```python
from build123d import *

# Parameters (mm, degrees)
F7_W      = 30
F7_H      = 30
F8_DEPTH  = 1700
F15_DEPTH = 15
F17_DEPTH = 15
F19_DEPTH = 15
F21_DEPTH = 15


with BuildPart() as f8:
    # F7 (on Top) → F8 (new body)
    with BuildSketch(Plane.XY):
        with Locations((-500, -15)):
            Rectangle(F7_W, F7_H)
    extrude(amount=F8_DEPTH)



with BuildPart() as f8b:
    # F7 (on Top) → F8, piece 2 (new body)
    with BuildSketch(Plane.XY):
        with Locations((500, -15)):
            Rectangle(F7_W, F7_H)
    extrude(amount=F8_DEPTH)


with BuildPart() as f8_1:
    add(f8.part)

    add(f8b.part)  # F15 merges F8b
    # F14 (on offset) → F15 (join)
    with BuildSketch(Plane.XY.offset(450)):
        with BuildLine():
            Line((485, 0), (0, 0))
            Line((0, 0), (-485, 0))
            Line((-485, 0), (-485, -30))
            Line((-485, -30), (-515, -30))
            Line((-515, -30), (-515, 0))
            Line((-515, 0), (-650, 0))
            Line((-650, 0), (-650, -360))
            ThreePointArc((-650, -360), (-638.2842712475, -388.2842712475), (-610, -400))
            Line((-610, -400), (0, -400))
            Line((0, -400), (610, -400))
            ThreePointArc((610, -400), (638.2842712475, -388.2842712475), (650, -360))
            Line((650, -360), (650, 0))
            Line((650, 0), (515, 0))
            Line((515, 0), (515, -30))
            Line((515, -30), (485, -30))
            Line((485, -30), (485, 0))
        make_face()
    extrude(amount=-F15_DEPTH)

    # F16 (on offset) → F17 (join)
    with BuildSketch(Plane.XY.offset(750)):
        with BuildLine():
            Line((0, -400), (610, -400))
            ThreePointArc((610, -400), (638.2842712475, -388.2842712475), (650, -360))
            Line((650, -360), (650, 0))
            Line((650, 0), (515, 0))
            Line((515, 0), (515, -30))
            Line((515, -30), (485, -30))
            Line((485, -30), (485, 0))
            Line((485, 0), (0, 0))
            Line((0, 0), (-485, 0))
            Line((-485, 0), (-485, -30))
            Line((-485, -30), (-515, -30))
            Line((-515, -30), (-515, 0))
            Line((-515, 0), (-650, 0))
            Line((-650, 0), (-650, -360))
            ThreePointArc((-650, -360), (-638.2842712475, -388.2842712475), (-610, -400))
            Line((-610, -400), (0, -400))
        make_face()
    extrude(amount=-F17_DEPTH)

    # F18 (on offset) → F19 (join)
    with BuildSketch(Plane.XY.offset(1150)):
        with BuildLine():
            Line((0, -400), (610, -400))
            ThreePointArc((610, -400), (638.2842712475, -388.2842712475), (650, -360))
            Line((650, -360), (650, 0))
            Line((650, 0), (515, 0))
            Line((515, 0), (515, -30))
            Line((515, -30), (485, -30))
            Line((485, -30), (485, 0))
            Line((485, 0), (0, 0))
            Line((0, 0), (-485, 0))
            Line((-485, 0), (-485, -30))
            Line((-485, -30), (-515, -30))
            Line((-515, -30), (-515, 0))
            Line((-515, 0), (-650, 0))
            Line((-650, 0), (-650, -360))
            ThreePointArc((-650, -360), (-638.2842712475, -388.2842712475), (-610, -400))
            Line((-610, -400), (0, -400))
        make_face()
    extrude(amount=-F19_DEPTH)

    # F20 (on offset) → F21 (join)
    with BuildSketch(Plane.XY.offset(1550)):
        with BuildLine():
            Line((0, -400), (610, -400))
            ThreePointArc((610, -400), (638.2842712475, -388.2842712475), (650, -360))
            Line((650, -360), (650, 0))
            Line((650, 0), (515, 0))
            Line((515, 0), (515, -30))
            Line((515, -30), (485, -30))
            Line((485, -30), (485, 0))
            Line((485, 0), (0, 0))
            Line((0, 0), (-485, 0))
            Line((-485, 0), (-485, -30))
            Line((-485, -30), (-515, -30))
            Line((-515, -30), (-515, 0))
            Line((-515, 0), (-650, 0))
            Line((-650, 0), (-650, -360))
            ThreePointArc((-650, -360), (-638.2842712475, -388.2842712475), (-610, -400))
            Line((-610, -400), (0, -400))
        make_face()
    extrude(amount=-F21_DEPTH)


solid = f8_1.part
```
Geometry: final body of the model. Coordinates: model frame, mm. Give positions to 0.01 mm unless a question says otherwise; leave off trailing zeros. Order: outer loops, then holes, each group sorted by start corner. A loop starts at its lowest first (then second) coordinate and runs counter-clockwise, first axis right, second up. Notation, with made-up numbers: (33.25, 54) -> (38.25, 54) arc R16 ccw to (38.25, 62) -> close; hole circle Ø3 at (89, 34). An arc over 180 degrees is marked (long way). Write each question's results on one line, items separated by ' | '. Start each with the question number.
1) Section B-B (y = -97.5). Return loops of the section in (x, z).
2) Line query: line 1 (Z direction, x = -59, y = -298); line 2 (Y direction, x = -491.5, z = 1132.5). Output: solid intervals per line, ascending. Write a range as from..to.
3) Section A-A (x = -296). Return loops of the section in (y, z).
4) Section C-C (z = 1450.5). Return loops of the section in (x, y), then the cut area to 3 significant figures.
5) Draft query along Z for faces 1 (the flat face through (-9, -197, 1150)), 2 (the flat face through (-3, 0, 1539)). Return one class per face: pulls with the +Z half, pulls with the -Z half, needs draft (parallel to the pull), parting line crosses it, or undercut.
6) First-contact query: pin 1 (9 mm diameter, centred on y = -15.5, z = 271.5, fed in from +X); pin 2 (24 mm diameter, centred on x = 493, z = 525.5, fed in from -Y); pin 3 (9 mm diameter, centred on y = -11.5, z = 995.5, fed in from -X). Flat tips, straight axial feed; report the tip coordinate or a pass-through.
Calculated:
1) outline: (-650, 435) -> (650, 435) -> (650, 450) -> (-650, 450) -> close; (-650, 735) -> (650, 735) -> (650, 750) -> (-650, 750) -> close; (-650, 1135) -> (650, 1135) -> (650, 1150) -> (-650, 1150) -> close; (-650, 1535) -> (650, 1535) -> (650, 1550) -> (-650, 1550) -> close
2) line 1: 435..450, 735..750, 1135..1150, 1535..1550 | line 2: -30..0
3) outline: (-400, 435) -> (0, 435) -> (0, 450) -> (-400, 450) -> close; (-400, 735) -> (0, 735) -> (0, 750) -> (-400, 750) -> close; (-400, 1135) -> (0, 1135) -> (0, 1150) -> (-400, 1150) -> close; (-400, 1535) -> (0, 1535) -> (0, 1550) -> (-400, 1550) -> close
4) outline: (-515, -30) -> (-485, -30) -> (-485, 0) -> (-515, 0) -> close; (485, -30) -> (515, -30) -> (515, 0) -> (485, 0) -> close | area: 1,800 mm2
5) face 1: undercut | face 2: needs draft
6) pin 1: x = 515 | pin 2: y = -30 | pin 3: x = -515
